For this review, take the finished solid that the model builds, in its own axes (mm). Face numbers are marked on the shaded views. A direction names the side the tool comes from. Round coordinates to 2 decimals unless told otherwise and drop trailing zeros. Loops run counter-clockwise (first coordinate to the right, second up) from the corner with the lowest first, then second, coordinate; pieces in that order, holes last.
1. Consider section A-A on x = 17. State the section outline as (y, z) points.
2. Draft analysis for pull direction X (two halves, no side actions). For the marked faces 4, 5, 6 and 7, state which applies: released by +X, released by -X, zero draft, split by the parting line, or undercut.
3. To check wall thickness, follow line 1 along Z through (x, y) = (9, 10.5); line 2 along Z through (x, y) = (20.5, 1.5); line 3 along X through (y, z) = (9.5, -8). State the ranges of each line that lie inside material, in increasing order.
4. Consider section C-C on y = 18. State the section outline as (x, z) points.
5. Consider section D-D on z = -12. State the section outline as (x, y) points.
6. Tool access review of the marked faces 1, 2 and 3: name each direction out of +Z, -Z, +X, -X, +Y, -Y from which nothing blocks a thin tool from reaching the whole face with its end or side.
7. Clearance check with flat-ended pins moving along their axes: pin 1 Ø1 at (x, z) = (9, 5) entering from +Y; pin 2 Ø1 at (x, z) = (-1, -1) entering from -Y; pin 3 Ø1.6 at (y, z) = (-1, 0.5) entering from +X. State where each tip first meets the part, or that it passes through.
8. Consider section B-B on z = 0. State how many separate pieces and enclosed holes the cut face has, then the cut area to 3 significant figures.
Autodesk Inventor part; units mm, degrees
ref_plane "Work Plane1" through (0, 0, -11) normal (-0.7071, 0.7071, 0) x (0, 0, -1)
ref_plane "Work Plane2" through (0, 0, 0) normal (0, 0, 1) x (1, 0, 0)
ref_plane "YZ Plane" through (0, 0, 0) normal (1, 0, 0) x (0, 1, 0)
sketch "Sketch1" plane through (0, 0, 0) normal (0, 0, 1) x (1, 0, 0)
  line L0 (0, 0) -> (0, 35)
  line L1 (0, 35) -> (4, 35)
  line L2 (4, 35) -> (4, 4)
  line L3 (4, 4) -> (35, 4)
  line L4 (35, 4) -> (35, 0)
  line L5 (35, 0) -> (0, 0)
  dimension "d8" = 35
  dimension "d10" = 4
  dimension "d11" = 4
  dimension "d12" = 35
extrude "Extrusion1" add sketch "Sketch1" along normal blind 11 and the other way blind 11
ref_plane "Work Plane1" through (0, 0, -11) normal (-0.7071, 0.7071, 0) x (0, 0, -1)
sketch "Sketch2" plane through (4, 4, -11) normal (1, 0, 0) x (0, 0, -1)
  line L0 (-11, 21.9) -> (-11, 6.1) construction
  line L1 (-14.4, 18.5) -> (-14.4, 9.5)
  line L2 (-7.6, 9.5) -> (-7.6, 18.5)
  arc A0 (-7.6, 18.5) -> (-14.4, 18.5) centre (-11, 18.5) ccw
  arc A1 (-14.4, 9.5) -> (-7.6, 9.5) centre (-11, 9.5) ccw
  line L3 (0, 0) -> (-22, 0)
  line L4 (-22, -4) -> (-11, -4)
  line L5 (-22, 0) -> (-22, 31)
  point P0 (-11, 14)
  dimension "d16" = 6.8
  dimension "d17" = 9
  dimension "d19" = 13.5
  dimension "d28" = 11
extrude "Extrusion2" cut sketch "Sketch2" against normal up to surface (4 mm away)
mirror "Mirror1" about plane through (0, 0, -11) normal (-0.7071, 0.7071, 0) of "Extrusion2"
sketch "Sketch3" plane through (0, 0, 11) normal (0, 0, 1) x (1, 0, 0)
  line L0 (4, 35) -> (0, 35)
  line L1 (0, 35) -> (6.5, 35)
  line L2 (6.5, 35) -> (6.5, 29.7)
  line L3 (35, 0) -> (35, 4)
  line L4 (35, 0) -> (35, 6.5)
  line L5 (35, 6.5) -> (29.7, 6.5)
  line L6 (29.7, 6.5) -> (6.5, 29.7)
  line L7 (0, 35) -> (0, 0)
  line L8 (0, 35) -> (0, 0)
  line L9 (0, 0) -> (35, 0)
  dimension "d22" = 6.5
  dimension "d23" = 5.3
  dimension "d24" = 6.5
  dimension "d25" = 5.3
ref_plane "Work Plane2" through (0, 0, 0) normal (0, 0, 1) x (1, 0, 0)
extrude "Extrusion3" add sketch "Sketch3" along normal blind 3
mirror "Mirror2" about plane through (0, 0, 0) normal (0, 0, 1) of "Extrusion3"
fillet "Fillet1" radius 0.5 6 edges at (35, 6.5, 12.5) (35, 6.5, -12.5) (6.5, 35, -12.5) (6.5, 35, 12.5) (35, 4, 0) (4, 35, 0)
sketch "Sketch4" plane through (0, 0, 14) normal (0, -1, 0) x (1, 0, 0)
  line L0 (35, -3) -> (35, -25)
  line L1 (35, -14) -> (0, -14) construction
  line L2 (4.5, -11.2) -> (2.5, -11.2)
  line L3 (2.5, -11.2) -> (2.5, -16.8)
  line L4 (2.5, -16.8) -> (4.5, -16.8)
  line L5 (4.5, -16.8) -> (4.5, -11.2)
  line L6 (4.5, -11.2) -> (2.5, -16.8) construction
  line L7 (2.5, -11.2) -> (4.5, -16.8) construction
  line L8 (0, -28) -> (0, 0)
  line L9 (30.5, -11.2) -> (32.5, -11.2)
  line L10 (32.5, -11.2) -> (32.5, -16.8)
  line L11 (32.5, -16.8) -> (30.5, -16.8)
  line L12 (30.5, -16.8) -> (30.5, -11.2)
  line L13 (30.5, -11.2) -> (32.5, -16.8) construction
  line L14 (32.5, -11.2) -> (30.5, -16.8) construction
  point P0 (3.5, -14)
  point P1 (31.5, -14)
  dimension "d34" = 2
  dimension "d35" = 5.6
  dimension "d36" = 2.5
  dimension "d37" = 5.6
  dimension "d38" = 2
  dimension "d39" = 2.5
extrude "Extrusion4" add sketch "Sketch4" along normal blind 2
mirror "Mirror3" about plane through (0, 0, -11) normal (-0.7071, 0.7071, 0) of "Extrusion4"
properties part number "L Angle Bracket 30x30 31082023"
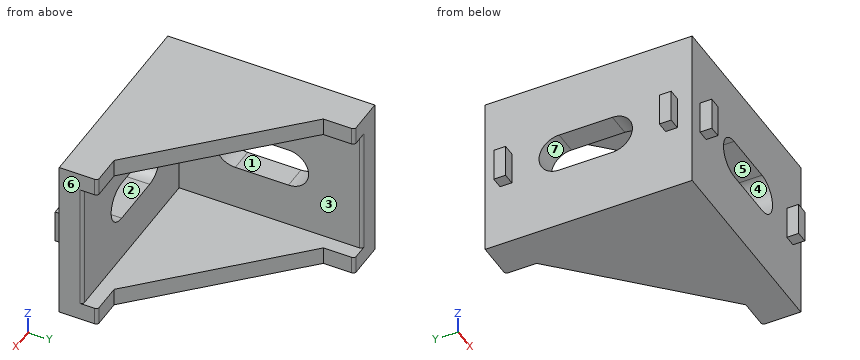
Resolved:
1. outline: (0, -14) - (19.2, -14) - (19.2, -11) - (4, -11) - (4, -3.4) - (0, -3.4) - close; (0, 3.4) - (4, 3.4) - (4, 11) - (19.2, 11) - (19.2, 14) - (0, 14) - close
2. face 4: undercut
2. face 5: undercut
2. face 6: released by +X
2. face 7: zero draft
3. line 1: z = -14 to -11, 11 to 14
3. line 2: z = -14 to -3.4, 3.4 to 14
3. line 3: x = 0 to 4
4. outline: (0, -14) - (18.2, -14) - (18.2, -11) - (4, -11) - (4, -3.4) - (0, -3.4) - close; (0, 3.4) - (4, 3.4) - (4, 11) - (18.2, 11) - (18.2, 14) - (0, 14) - close
5. outline: (0, 0) - (35, 0) - (35, 6) arc R0.5 ccw to (34.5, 6.5) - (29.7, 6.5) - (6.5, 29.7) - (6.5, 34.5) arc R0.5 ccw to (6, 35) - (0, 35) - close
6. face 1: +X, -X
6. face 2: +Y, -Y
6. face 3: +X, +Y
7. pin 1: stops at y = 4
7. pin 2: stops at y = 2.5
7. pin 3: stops at x = 32.5
8. separate pieces: 3
8. enclosed holes: 0
8. area: 153 mm2
